```python
from build123d import *

# Parameters (mm, degrees)
SKETCH_1_W          = 38
SKETCH_1_H          = 38
EXTRUDE_1_DEPTH     = 3
SKETCH_2_R          = 2.25
CUT_EXTRUDE_1_DEPTH = 28.531799796
SKETCH_3_R          = 2.75
SKETCH_3_R_2        = 7
CUT_EXTRUDE_2_DEPTH = 28.531799796
FILLET_1_R          = 3


with BuildPart() as part:
    # 草图1 → 凸台-拉伸1 (new, symmetric)
    with BuildSketch(Plane(origin=(0, 0, 0), x_dir=(1, 0, 0), z_dir=(0, 1, 0))):
        Rectangle(SKETCH_1_W, SKETCH_1_H)
    extrude(amount=EXTRUDE_1_DEPTH, both=True)

    # 草图2 → 切除-拉伸1 (cut, through all)
    with BuildSketch(Plane(origin=(0, 3, 0), x_dir=(1, 0, 0), z_dir=(0, 1, 0))):
        with Locations(Location((-14.5, 14.5, 0), (0, 0, 270))):
            Circle(SKETCH_2_R)
        with Locations(Location((-14.5, -14.5, 0), (0, 0, 90))):
            Circle(SKETCH_2_R)
        with Locations(Location((14.5, -14.5, 0), (0, 0, 270))):
            Circle(SKETCH_2_R)
        with Locations(Location((14.5, 14.5, 0), (0, 0, 90))):
            Circle(SKETCH_2_R)
    extrude(amount=-CUT_EXTRUDE_1_DEPTH, mode=Mode.SUBTRACT)

    # 草图3 → 切除-拉伸2 (cut, through all)
    with BuildSketch(Plane(origin=(0, 3, 0), x_dir=(1, 0, 0), z_dir=(0, 1, 0))):
        with Locations(Location((-8.308504679, 8.308504679, 0), (0, 0, 270))):
            Circle(SKETCH_3_R)
        with Locations(Location((-8.308504679, -8.308504679, 0), (0, 0, 90))):
            Circle(SKETCH_3_R)
        with Locations(Location((8.308504679, -8.308504679, 0), (0, 0, 270))):
            Circle(SKETCH_3_R)
        with Locations(Location((8.308504679, 8.308504679, 0), (0, 0, 90))):
            Circle(SKETCH_3_R)
        with Locations(Location((0, 0, 0), (0, 0, 270))):
            Circle(SKETCH_3_R_2)
    extrude(amount=-CUT_EXTRUDE_2_DEPTH, mode=Mode.SUBTRACT)

    # 圆角1
    fillet_1_edges = [part.edges().sort_by_distance(p)[0] for p in [
        (-19, 0, -19),
        (19, 0, -19),
        (19, 0, 19),
        (-19, 0, 19),
    ]]
    fillet(fillet_1_edges, radius=FILLET_1_R)


solid = part.part
```
Could you check a few things on this model? Use its own coordinates, in mm. Give positions to 0.01 mm unless a question says otherwise; leave off trailing zeros. Loops run counter-clockwise (first coordinate to the right, second up) from the corner with the lowest first, then second, coordinate; pieces in that order, holes last. Notation, with made-up numbers: (-23.75, 35.25) - (22.25, 35.25) arc R21 ccw to (22.25, 67.25) - close; hole circle Ø7 at (49.25, -12.5). An arc over 180 degrees is marked (long way). Answer in a Markdown table with one row per item. Add a question column.
Q1. If we section it at D-D (z = 14): List the corners of the cut face in (x, y) for me, plus the area to 3 significant figures.
Q2. If we section it at A-A (x = -14.5): List the corners of the cut face in (y, z) for me.
Q3. Please list where these lines run through material, in increasing order: L1, parallel to X at y = 1.55, z = -8.5; L2, parallel to X at y = -0.85, z = 14.5. Write a range as from..to.
Q4. If we section it at B-B (x = 0): List the corners of the cut face in (y, z) for me.
Q5. We'd pull the mould along X, two halves only. Please class faces 1 (the face through (5.624, 0.042, 7.712)), 2 (the face through (19, 0, 0)), 3 (the face through (0, 3, 8)): +X half, -X half, draft (parallel to the pull), parting line (faces both ways), or undercut.
Q6. If we section it at C-C (z = 0): List the corners of the cut face in (x, y) for me, plus the area to 3 significant figures.
The answers:
| question | item | result |
|---|---|---|
| 1 | outline | (-19, -3) - (-16.69, -3) - (-16.69, 3) - (-19, 3) - close; (-12.31, -3) - (12.31, -3) - (12.31, 3) - (-12.31, 3) - close; (16.69, -3) - (19, -3) - (19, 3) - (16.69, 3) - close |
| 1 | area | 175 mm^2 |
| 2 | outline | (-3, -19) - (3, -19) - (3, -16.75) - (-3, -16.75) - close; (-3, -12.25) - (3, -12.25) - (3, 12.25) - (-3, 12.25) - close; (-3, 16.75) - (3, 16.75) - (3, 19) - (-3, 19) - close |
| 3 | L1 | x = -19..-11.05, -5.57..5.57, 11.05..19 |
| 3 | L2 | x = -19..-16.75, -12.25..12.25, 16.75..19 |
| 4 | outline | (-3, -19) - (3, -19) - (3, -7) - (-3, -7) - close; (-3, 7) - (3, 7) - (3, 19) - (-3, 19) - close |
| 5 | face 1 | undercut |
| 5 | face 2 | +X half |
| 5 | face 3 | draft |
| 6 | outline | (-19, -3) - (-7, -3) - (-7, 3) - (-19, 3) - close; (7, -3) - (19, -3) - (19, 3) - (7, 3) - close |
| 6 | area | 144 mm^2 |
